```python
from build123d import *

# Parameters (mm, degrees)
F0_R     = 13.1445
F1_DEPTH = 4.826
F2_R     = 13.1445
F2_R_2   = 12.4206
F3_DEPTH = 1.524


# Not quite as in the source:
# - a fillet or chamfer that OpenCascade refuses, or shapes differently, is made with other operations: its cross-section is extruded or revolved along the edge and cut away or added


with BuildPart() as f1:
    # F0 (on Top) → F1 (new body)
    with BuildSketch(Plane.XY):
        Circle(F0_R)
    extrude(amount=F1_DEPTH)

    # F2 (on face) → F3 (join)
    with BuildSketch(Plane.XY.offset(4.826)):
        Circle(F2_R)
        Circle(F2_R_2, mode=Mode.SUBTRACT)
    extrude(amount=F3_DEPTH)

    # F4: chamfer of 0.762 on 1 edges, made by hand

    # F4_s1 → F4_t2 (revolve, cut)
    with BuildSketch(Plane.XZ):
        Polygon((13.1826, 6.35), (12.4206, 5.588), (12.4206, 6.35), align=None)
    revolve(axis=Axis((0, 0, 6.35), (0, 0, 1)), mode=Mode.SUBTRACT)


solid = f1.part
```
Can you work these out from the model? Positions are in its coordinate system, mm. Round coordinates to 2 decimals unless told otherwise and drop trailing zeros. Loops run counter-clockwise (first coordinate to the right, second up) from the corner with the lowest first, then second, coordinate; pieces in that order, holes last. Notation, with made-up numbers: (-28, 60.25) -> (20, 60.25) arc R37 ccw to (20, 97.25) -> close; hole circle Ø3 at (8.25, 41). An arc over 180 degrees is marked (long way). One line per item, written item: value. Start each with the question number.
1. If we section it at C-C, the plane z = 2: Write out the boundary of the cut face in (x, y), then the cut area to 3 significant figures.
2. For pin 1 (8 mm diameter, centred on x = -7, y = 0.5, fed in from -Z); pin 2 (3 mm diameter, centred on y = 4.5, z = 5, fed in from -X); pin 3 (2 mm diameter, centred on x = 2, y = -8.5, fed in from +Z), each with a flat end and sliding along its axis, tell me the tip position at first contact or that it passes through.
3. If we section it at A-A, the plane y = 0: Write out the boundary of the cut face in (x, z), then the cut area to 3 significant figures.
4. If I drill on probe 1 along Y at (x, z) = (0, 5.4); probe 2 along Z at (x, y) = (0.5, -9); probe 3 along X at (y, z) = (6.5, 5.75), over which ranges is the centre line in solid material (lowest first)?
5. If we mould it in two halves opening along Y, with no side actions, what happens to faces 1 (the flat face through (0, 0, 0)), 2 (the cylindrical face through (12.538, 3.948, 3.112)), 3 (the cylindrical face through (11.847, 3.731, 5.202))? For each: pulls with the +Y half, pulls with the -Y half, needs draft (parallel to the pull), parting line crosses it, or undercut.
Calculated:
1. outline: circle Ø26.29 at (0, 0)
1. area: 543 mm²
2. pin 1: stops at z = 0
2. pin 2: stops at x = -12.8
2. pin 3: stops at z = 4.83
3. outline: (-13.14, 0) -> (13.14, 0) -> (13.14, 6.31) -> (12.42, 5.59) -> (12.42, 4.83) -> (-12.42, 4.83) -> (-12.42, 5.59) -> (-13.14, 6.31) -> close
3. area: 128 mm²
4. probe 1: y = -13.14 to -12.42, 12.42 to 13.14
4. probe 2: z = 0 to 4.83
4. probe 3: x = -11.42 to -10.77, 10.77 to 11.42
5. face 1: needs draft
5. face 2: parting line crosses it
5. face 3: undercut
